Part model, mm, in its own coordinate system. Face numbers are marked on the shaded views. A direction names the side the tool comes from. Round coordinates to 2 decimals unless told otherwise and drop trailing zeros. Loops run counter-clockwise (first coordinate to the right, second up) from the corner with the lowest first, then second, coordinate; pieces in that order, holes last. Notation, with made-up numbers: M 60,-32.5 L 96,-32.5 A16 cw 96,-3.5 Z; hole C -4.75,16.25 d4. An arc over 180 degrees is marked long. Put each result on its own line as item: value. Start each with the question number.
1) Slice it at C-C on z = -8. Give the cut face in (x, y) (3 decimals), then the cut area to 3 significant figures.
2) Which spindle directions (+Z, -Z, +X, -X, +Y, -Y) get a long thin tool onto all of the face, cutting with end or side? Do the marked faces 1, 2, 3, 4 and 5. Say none if no direction does.
3) Slice it at D-D on x = -13. Give the cut face in (y, z) (3 decimals).
4) Slice it at B-B on z = 87. Give the cut face in (x, y).
5) Probe line 1 along X through (y, z) = (11.5, 7) (3 decimals); line 2 along X through (y, z) = (-10, 15) (3 decimals); line 3 along Y through (x, z) = (35, 0) (3 decimals). List the from-to ranges inside material, lowest first.
6) Pull direction Z, two halves, no side cores. Call the marked faces 6, 7 and 8: +Z half, -Z half, draft (parallel to the pull), parting line (faces both ways), or undercut.
7) Drop flat-ended pins along their axis: pin 1 Ø12 at (y, z) = (-18, 29) entering from -X (3 decimals); pin 2 Ø22 at (x, z) = (-0.02, 75.95) entering from -Y; pin 3 Ø21 at (x, y) = (4, -2.5) entering from -Z; pin 4 Ø3 at (x, z) = (-7, 54) entering from +Y. Give the stop position or say it passes through.
8) Slice it at A-A on y = 0. Give the cut face in (x, z) (3 decimals), then the cut area to 3 significant figures.
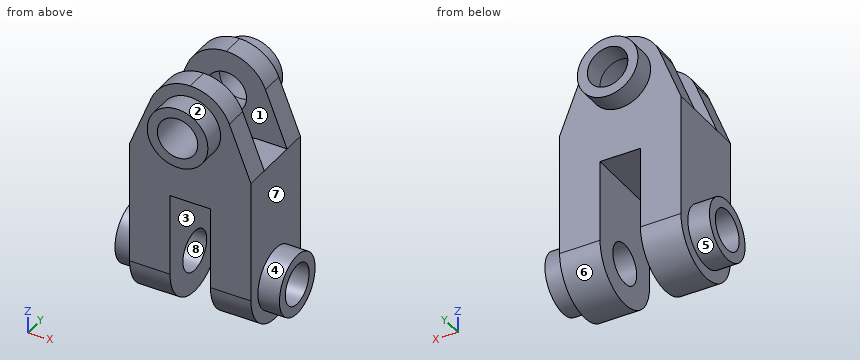
```python
from build123d import *

# Parameters (mm, degrees)
SKETCH3_W           = 38.1
SKETCH3_H           = 10.668
BOSS_EXTRUDE1_DEPTH = 28.575
SKETCH4_W           = 19.05
SKETCH4_H           = 38.608
SKETCH4_H_2         = 19.812
SKETCH4_R           = 9.525
CUT_EXTRUDE1_DEPTH  = 40.624
SKETCH5_R           = 14.2875
SKETCH5_R_2         = 9.525
BOSS_EXTRUDE2_DEPTH = 10.16
BOSS_EXTRUDE3_START = -39.624
SKETCH5_3_R         = 14.2875
SKETCH5_3_R_2       = 9.525
BOSS_EXTRUDE3_DEPTH = 10.16
SKETCH6_R           = 9.525
CUT_EXTRUDE2_DEPTH  = 58.15
SKETCH7_R           = 14.25575
SKETCH7_R_2         = 9.525
BOSS_EXTRUDE4_DEPTH = 10.16
BOSS_EXTRUDE5_START = -57.15
SKETCH7_2_R         = 14.25575
SKETCH7_2_R_2       = 9.525
BOSS_EXTRUDE5_DEPTH = 10.16


with BuildPart() as part:
    # Sketch3 → Boss-Extrude1 (new body, symmetric)
    with BuildSketch(Plane(origin=(0, 0, 0), x_dir=(0, 0, -1), z_dir=(1, 0, 0))):
        with BuildLine():
            ThreePointArc((0, -19.812), (19.812, 0), (0, 19.812))
            Line((0, 19.812), (-57.658, 19.812))
            Line((-57.658, 19.812), (-57.658, 9.144))
            Line((-57.658, 9.144), (-57.658, -9.144))
            Line((-57.658, -9.144), (-57.658, -19.812))
            Line((-57.658, -19.812), (0, -19.812))
        make_face()
        with Locations((-76.708, 14.478)):
            Rectangle(SKETCH3_W, SKETCH3_H)
        with Locations((-76.708, -14.478)):
            Rectangle(SKETCH3_W, SKETCH3_H)
    extrude(amount=BOSS_EXTRUDE1_DEPTH, both=True)

    # Sketch4 → Cut-Extrude1 (cut, through all)
    with BuildSketch(Plane(origin=(0, 19.812, 0), x_dir=(1, 0, 0), z_dir=(0, 1, 0))):
        with Locations((0, -19.304)):
            Rectangle(SKETCH4_W, SKETCH4_H)
        with Locations((0, 9.906)):
            Rectangle(SKETCH4_W, SKETCH4_H_2)
        with BuildLine():
            Line((28.575, -95.758), (28.575, -57.658))
            Line((28.575, -57.658), (18.395099317, -83.264992565))
            ThreePointArc((18.395099317, -83.264992565), (11.109122589, -92.339889472), (-0.015432736, -95.758))
            Line((-0.015432736, -95.758), (28.575, -95.758))
        make_face()
        with Locations((-0.015432773, -75.946)):
            Circle(SKETCH4_R)
        with BuildLine():
            Line((-18.433578911, -83.24581074), (-28.575, -57.658))
            Line((-28.575, -57.658), (-28.575, -95.758))
            Line((-28.575, -95.758), (-0.015432736, -95.758))
            ThreePointArc((-0.015432736, -95.758), (-11.148525176, -92.334093164), (-18.433578911, -83.24581074))
        make_face()
    extrude(amount=-CUT_EXTRUDE1_DEPTH, mode=Mode.SUBTRACT)

    # Sketch5 → Boss-Extrude2 (add)
    with BuildSketch(Plane(origin=(0, 19.812, 0), x_dir=(1, 0, 0), z_dir=(0, 1, 0))):
        with Locations((-0.015432773, -75.946)):
            Circle(SKETCH5_R)
        with Locations((-0.015432773, -75.946)):
            Circle(SKETCH5_R_2, mode=Mode.SUBTRACT)
    extrude(amount=BOSS_EXTRUDE2_DEPTH)

    # Sketch5<3> → Boss-Extrude3 (add)
    with BuildSketch(Plane(origin=(0, 19.812, 0), x_dir=(1, 0, 0), z_dir=(0, 1, 0)).offset(BOSS_EXTRUDE3_START)):
        with Locations((-0.015432773, -75.946)):
            Circle(SKETCH5_3_R)
        with Locations((-0.015432773, -75.946)):
            Circle(SKETCH5_3_R_2, mode=Mode.SUBTRACT)
    extrude(amount=-BOSS_EXTRUDE3_DEPTH)

    # Sketch6 → Cut-Extrude2 (cut, through all)
    with BuildSketch(Plane(origin=(28.575, 0, 0), x_dir=(0, 0, -1), z_dir=(1, 0, 0))):
        Circle(SKETCH6_R)
    extrude(amount=-CUT_EXTRUDE2_DEPTH, mode=Mode.SUBTRACT)

    # Sketch7 → Boss-Extrude4 (add)
    with BuildSketch(Plane(origin=(28.575, 0, 0), x_dir=(0, 0, -1), z_dir=(1, 0, 0))):
        Circle(SKETCH7_R)
        Circle(SKETCH7_R_2, mode=Mode.SUBTRACT)
    extrude(amount=BOSS_EXTRUDE4_DEPTH)

    # Sketch7<2> → Boss-Extrude5 (add)
    with BuildSketch(Plane(origin=(28.575, 0, 0), x_dir=(0, 0, -1), z_dir=(1, 0, 0)).offset(BOSS_EXTRUDE5_START)):
        Circle(SKETCH7_2_R)
        Circle(SKETCH7_2_R_2, mode=Mode.SUBTRACT)
    extrude(amount=-BOSS_EXTRUDE5_DEPTH)


solid = part.part
```
Recorded:
1. outline: M -38.735,-11.799 L -28.575,-11.799 L -28.575,-18.125 L -9.525,-18.125 L -9.525,-5.17 L -38.735,-5.17 Z; M -38.735,5.17 L -9.525,5.17 L -9.525,18.125 L -28.575,18.125 L -28.575,11.799 L -38.735,11.799 Z; M 9.525,-18.125 L 28.575,-18.125 L 28.575,-11.799 L 38.735,-11.799 L 38.735,-5.17 L 9.525,-5.17 Z; M 9.525,5.17 L 38.735,5.17 L 38.735,11.799 L 28.575,11.799 L 28.575,18.125 L 9.525,18.125 Z
1. area: 1,260 mm2
2. face 1: +Z, +X, -X
2. face 2: -Y
2. face 3: -Z, +Y, -Y
2. face 4: +X
2. face 5: -X
3. outline: M -29.972,69.985 L -19.812,69.985 L -19.812,0 A19.812 ccw 19.812,0 L 19.812,69.985 L 29.972,69.985 L 29.972,81.907 L 19.812,81.907 L 19.812,90.91 L 9.144,90.91 L 9.144,57.658 L -9.144,57.658 L -9.144,90.91 L -19.812,90.91 L -19.812,81.907 L -29.972,81.907 Z; hole C 0,0 d19.05
4. outline: M -16.46,-19.81 L -9.07,-19.81 L -9.07,-29.97 L 9.04,-29.97 L 9.04,-19.81 L 16.43,-19.81 L 16.43,-9.14 L -16.46,-9.14 Z; M -16.46,9.14 L 16.43,9.14 L 16.43,19.81 L 9.04,19.81 L 9.04,29.97 L -9.07,29.97 L -9.07,19.81 L -16.46,19.81 Z
5. line 1: x = -38.735 to -9.525, 9.525 to 38.735
5. line 2: x = -28.575 to -9.525, 9.525 to 28.575
5. line 3: y = -14.256 to -9.525, 9.525 to 14.256
6. face 6: -Z half
6. face 7: draft
6. face 8: undercut
7. pin 1: stops at x = -28.575
7. pin 2: stops at y = -29.97
7. pin 3: stops at z = -19.81
7. pin 4: stops at y = 19.81
8. outline: M -38.735,-14.256 L -28.575,-14.256 L -28.575,-19.812 L -9.525,-19.812 L -9.525,-9.525 L -38.735,-9.525 Z; M -38.735,9.525 L -9.525,9.525 L -9.525,38.608 L 9.525,38.608 L 9.525,9.525 L 38.735,9.525 L 38.735,14.256 L 28.575,14.256 L 28.575,57.658 L -28.575,57.658 L -28.575,14.256 L -38.735,14.256 Z; M 9.525,-19.812 L 28.575,-19.812 L 28.575,-14.256 L 38.735,-14.256 L 38.735,-9.525 L 9.525,-9.525 Z
8. area: 2,780 mm2
